Print and shaded views of the part. All mm, measured from the part's lowest x, y and z. Round coordinates to 2 decimals unless told otherwise and drop trailing zeros. Order: outer loops, then holes, each group sorted by start corner. A loop starts at its lowest first (then second) coordinate and runs counter-clockwise, first axis right, second up. Notation, with made-up numbers: (33.25, 16) - (56.25, 16) arc R16 cw to (56.25, 24) - close; hole circle Ø2 at (43, -29). An arc over 180 degrees is marked (long way). Write item = value, one per line.
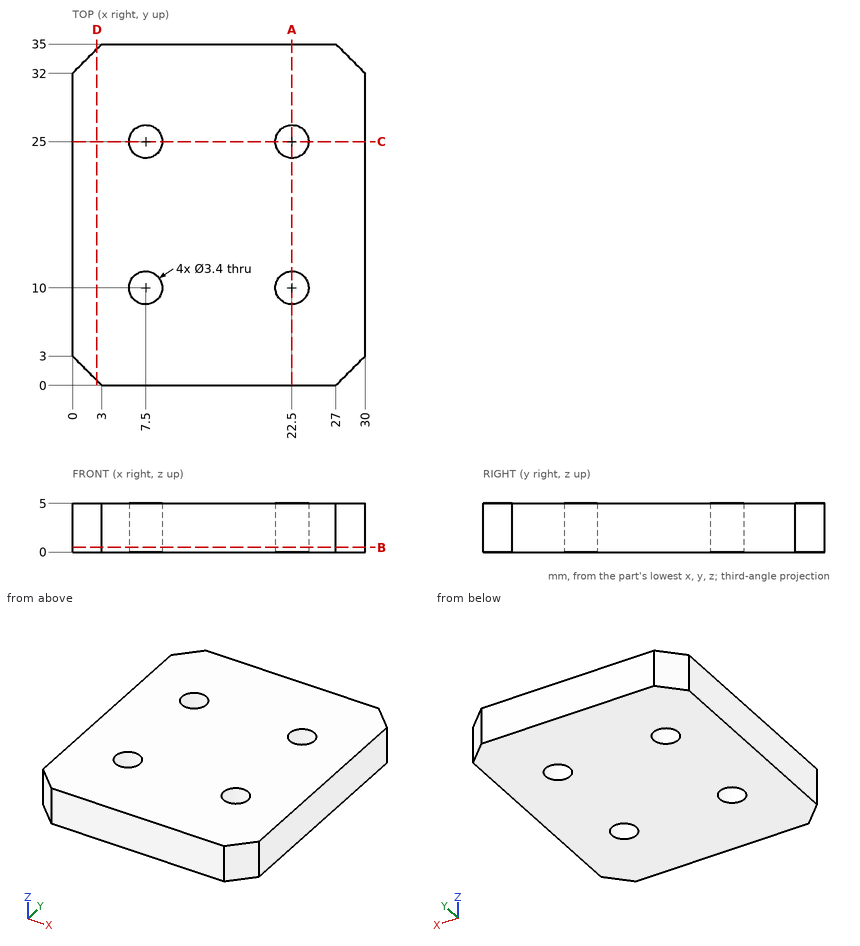
(1) Band-saw the part on A-A on x = 22.5. List the corners of the cut face in (y, z).
Solved:
outline = (0, 0) - (8.3, 0) - (8.3, 5) - (0, 5) - close; (11.7, 0) - (23.3, 0) - (23.3, 5) - (11.7, 5) - close; (26.7, 0) - (35, 0) - (35, 5) - (26.7, 5) - close
(2) Band-saw the part on C-C on y = 25. List the corners of the cut face in (x, z).
Solved:
outline = (0, 0) - (5.8, 0) - (5.8, 5) - (0, 5) - close; (9.2, 0) - (20.8, 0) - (20.8, 5) - (9.2, 5) - close; (24.2, 0) - (30, 0) - (30, 5) - (24.2, 5) - close
(3) Band-saw the part on D-D on x = 2.5. List the corners of the cut face in (y, z), plus the area to 3 significant figures.
Solved:
outline = (0.5, 0) - (34.5, 0) - (34.5, 5) - (0.5, 5) - close
area = 170 mm²
(4) Band-saw the part on B-B on z = 0.5. List the corners of the cut face in (x, y), plus the area to 3 significant figures.
Solved:
outline = (0, 3) - (3, 0) - (27, 0) - (30, 3) - (30, 32) - (27, 35) - (3, 35) - (0, 32) - close; hole circle Ø3.4 at (7.5, 10); hole circle Ø3.4 at (7.5, 25); hole circle Ø3.4 at (22.5, 10); hole circle Ø3.4 at (22.5, 25)
area = 996 mm²
(5) Probe line 1 along Y through (x, z) = (7.5, 3.95); line 2 along Y through (x, z) = (6.25, 2); line 3 along X through (y, z) = (24, 2.05). List the from-to ranges inside material, lowest first.
Solved:
line_1 = 0 to 8.3, 11.7 to 23.3, 26.7 to 35
line_2 = 0 to 8.85, 11.15 to 23.85, 26.15 to 35
line_3 = 0 to 6.13, 8.87 to 21.13, 23.87 to 30
